Check sheet for the modelled part. Datum: model origin and axes. Units: mm. Face numbers are marked on the shaded views. Round coordinates to 2 decimals unless told otherwise and drop trailing zeros. Order: outer loops, then holes, each group sorted by start corner. A loop starts at its lowest first (then second) coordinate and runs counter-clockwise, first axis right, second up.
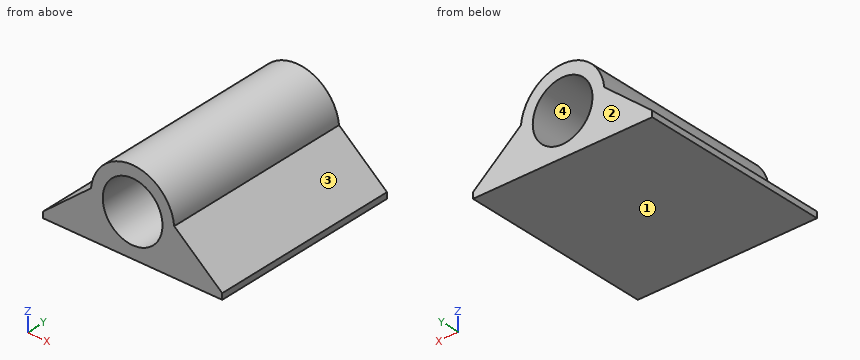
```python
from build123d import *

# Parameters (mm, degrees)
F0_R     = 2.5
F1_DEPTH = 16


with BuildPart() as f1:
    # F0 (on Front) → F1 (new body)
    with BuildSketch(Plane.XZ):
        with BuildLine():
            Line((-15, 0), (0, 0))
            Line((0, 0), (0, 0.5))
            Line((0, 0.5), (-4.016613, 3.870338))
            ThreePointArc((-4.016613, 3.870338), (-7.5, 7.029729), (-10.983387, 3.870338))
            Line((-10.983387, 3.870338), (-15, 0.5))
            Line((-15, 0.5), (-15, 0))
        make_face()
        with Locations((-7.5, 3.529729)):
            Circle(F0_R, mode=Mode.SUBTRACT)
    extrude(amount=F1_DEPTH)


solid = f1.part
```
Item 1: Sectioned sample at D-D (x = -12.75). Record the cut outline in (y, z), and give its area (3 significant figures).
Answer:
outline: (-16, 0) - (0, 0) - (0, 2.39) - (-16, 2.39) - close
area: 38.2 mm2
Item 2: Release check for a two-part mould opening along Z. For the marked faces 1, 2, 3 and 4 record: released by +Z, released by -Z, zero draft, split by the parting line, or undercut.
Answer:
face 1: released by -Z
face 2: zero draft
face 3: released by +Z
face 4: undercut
Item 3: Sectioned sample at B-B (y = -13.5). Record the cut outline in (x, z), and give its area (3 significant figures).
Answer:
outline: (-15, 0) - (0, 0) - (0, 0.5) - (-4.02, 3.87) arc R3.5 ccw to (-10.98, 3.87) - (-15, 0.5) - close; hole circle Ø5 at (-7.5, 3.53)
area: 41.7 mm2
Item 4: Sectioned sample at A-A (x = -7.5). Record the cut outline in (y, z), and give its area (3 significant figures).
Answer:
outline: (-16, 0) - (0, 0) - (0, 1.03) - (-16, 1.03) - close; (-16, 6.03) - (0, 6.03) - (0, 7.03) - (-16, 7.03) - close
area: 32.5 mm2
Item 5: Go/stop test with flat-tipped pins: P1, Ø5, axis at x = -5, y = -3, coming from the +Z side; P2, Ø1, axis at x = -9.5, y = -13, coming from the +Z side; P3, Ø3, axis at x = -7.5, z = 3.53, coming from the +Y side (3 decimals). Record where each tip stops, or that it passes through.
Answer:
P1: stops at z = 7.03
P2: stops at z = 6.69
P3: passes through
Item 6: Sectioned sample at C-C (z = 3.25). Record the cut outline in (x, y), and give its area (3 significant figures).
Answer:
outline: (-11.72, -16) - (-9.98, -16) - (-9.98, 0) - (-11.72, 0) - close; (-5.02, -16) - (-3.28, -16) - (-3.28, 0) - (-5.02, 0) - close
area: 55.6 mm2
Item 7: Scan lines: line 1 along Z through (x, y) = (-7.5, -3.25); line 2 along X through (y, z) = (-3.5, 1.5); line 3 along X through (y, z) = (-9.25, 2). Record each from-to range of solid material in increasing order.
Answer:
line 1: z = 0 to 1.03, 6.03 to 7.03
line 2: x = -13.81 to -8.96, -6.04 to -1.19
line 3: x = -13.21 to -9.48, -5.52 to -1.79
